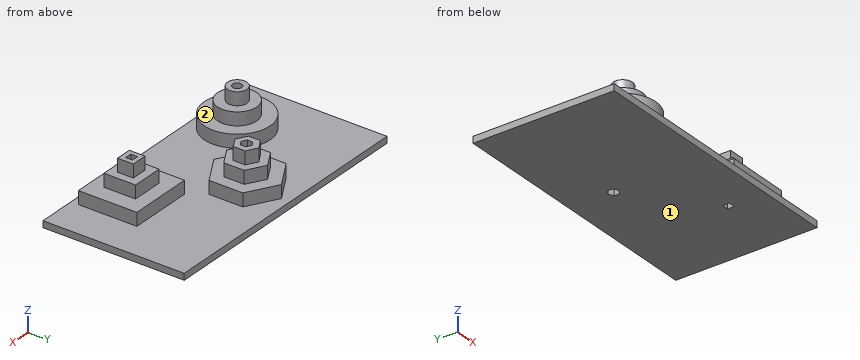
from build123d import *

# Parameters (mm, degrees)
SKETCH_R        = 50.540208
PAD_DEPTH       = 20
SKETCH001_R     = 30.027683
PAD001_DEPTH    = 20
SKETCH002_R     = 15.008606
PAD002_DEPTH    = 20
SKETCH003_R     = 7.050667
POCKET_DEPTH    = 60.001
SKETCH004_W     = 420.746094
SKETCH004_H     = 217.580834
PAD003_DEPTH    = 10
SKETCH005_W     = 98.75679
SKETCH005_H     = 90.115562
PAD004_DEPTH    = 20
SKETCH006_W     = 48.761093
SKETCH006_H     = 48.761156
PAD005_DEPTH    = 20
SKETCH007_W     = 24.319153
SKETCH007_H     = 24.30114
PAD006_DEPTH    = 20
SKETCH008_W     = 10.654495
SKETCH008_H     = 10.502288
POCKET001_DEPTH = 70.001
PAD007_DEPTH    = 20
PAD008_DEPTH    = 20
PAD009_DEPTH    = 20
POCKET002_DEPTH = 70.001


with BuildPart() as part:
    # Sketch → Pad (new body)
    with BuildSketch(Plane.XY):
        Circle(SKETCH_R)
    extrude(amount=PAD_DEPTH)

    # Sketch001 (on Face3 of Pad) → Pad001 (join)
    with BuildSketch(Plane.XY.offset(20)):
        Circle(SKETCH001_R)
    extrude(amount=PAD001_DEPTH)

    # Sketch002 (on Face5 of Pad001) → Pad002 (join)
    with BuildSketch(Plane.XY.offset(40)):
        Circle(SKETCH002_R)
    extrude(amount=PAD002_DEPTH)

    # Sketch003 (on Face7 of Pad002) → Pocket (cut, through all)
    with BuildSketch(Plane.XY.offset(60)):
        Circle(SKETCH003_R)
    extrude(amount=-POCKET_DEPTH, mode=Mode.SUBTRACT)

    # Sketch004 → Pad003 (join)
    with BuildSketch(Plane.XY):
        with Locations((116.873352, 52.568348)):
            Rectangle(SKETCH004_W, SKETCH004_H)
    extrude(amount=-PAD003_DEPTH)

    # Sketch005 (on Face4 of Pad003) → Pad004 (join)
    with BuildSketch(Plane.XY):
        with Locations((219.817588, 0.267387)):
            Rectangle(SKETCH005_W, SKETCH005_H)
    extrude(amount=PAD004_DEPTH)

    # Sketch006 (on Face13 of Pad004) → Pad005 (join)
    with BuildSketch(Plane.XY.offset(20)):
        with Locations((219.351036, -0.022332)):
            Rectangle(SKETCH006_W, SKETCH006_H)
    extrude(amount=PAD005_DEPTH)

    # Sketch007 (on Face20 of Pad005) → Pad006 (join)
    with BuildSketch(Plane.XY.offset(40)):
        with Locations((219.415116, -0.255952)):
            Rectangle(SKETCH007_W, SKETCH007_H)
    extrude(amount=PAD006_DEPTH)

    # Sketch008 (on Face27 of Pad006) → Pocket001 (cut, through all)
    with BuildSketch(Plane.XY.offset(60)):
        with Locations((219.071236, -0.040661)):
            Rectangle(SKETCH008_W, SKETCH008_H)
    extrude(amount=-POCKET001_DEPTH, mode=Mode.SUBTRACT)

    # Sketch009 (on Face4 of Pocket001) → Pad007 (join)
    with BuildSketch(Plane.XY):
        Polygon((152.636142, 69.881975), (152.636142, 121.928939), (107.562149, 147.952421), (62.488156, 121.928939), (62.488156, 69.881975), (107.562149, 43.858493), align=None)
    extrude(amount=PAD007_DEPTH)

    # Sketch010 (on Face24 of Pad007) → Pad008 (join)
    with BuildSketch(Plane.XY.offset(20)):
        Polygon((107.233368, 63.429135), (134.533937, 79.191126), (134.533937, 110.715108), (107.233368, 126.477099), (79.932799, 110.715108), (79.932799, 79.191126), align=None)
    extrude(amount=PAD008_DEPTH)

    # Sketch011 (on Face43 of Pad008) → Pad009 (join)
    with BuildSketch(Plane.XY.offset(40)):
        Polygon((107.227683, 76.060802), (123.144716, 85.250505), (123.144716, 103.629912), (107.227683, 112.819615), (91.31065, 103.629912), (91.31065, 85.250505), align=None)
    extrude(amount=PAD009_DEPTH)

    # Sketch012 (on Face52 of Pad009) → Pocket002 (cut, through all)
    with BuildSketch(Plane.XY.offset(60)):
        Polygon((107.152039, 85.588319), (114.400809, 89.773399), (114.400809, 98.143557), (107.152039, 102.328637), (99.903269, 98.143557), (99.903269, 89.773399), align=None)
    extrude(amount=-POCKET002_DEPTH, mode=Mode.SUBTRACT)


solid = part.part
Check sheet for the modelled part. Datum: model origin and axes. Units: mm. Face numbers are marked on the shaded views. Coordinates: 2 decimals unless noted, no trailing zeros. Loops run counter-clockwise (first coordinate to the right, second up) from the corner with the lowest first, then second, coordinate; pieces in that order, holes last. Notation, with made-up numbers: (10, 65.5) -> (51, 65.5) arc R6 ccw to (51, 71.5) -> close; hole circle Ø11 at (2, 4.25). An arc over 180 degrees is marked (long way). Write item = value, one per line. Start each with the question number.
1. Section check C-C on x = 157. Record the cut outline in (y, z), then the cut area to 3 significant figures.
2. Depth check by flat-ended pin: P1, Ø8, axis at y = 1.5, z = 17.5, coming from the -X side; P2, Ø22, axis at x = 219, z = 51.5, coming from the +Y side; P3, Ø6.5, axis at y = 96, z = 35.5, coming from the +X side. Enter the tip coordinate at first touch or a pass-through.
3. Draft check along X on the marked faces 1 and 2. Enter one of: released by +X, released by -X, zero draft, split by the parting line, or undercut.
4. Section check B-B on x = 0. Record the cut outline in (y, z).
5. Material ranges on line 1 (Y direction, x = 0, z = 14); line 2 (Y direction, x = 0, z = 33.5); line 3 (X direction, y = 45, z = 7) (3 decimals), recorded low to high.
6. Section check A-A on z = 33.5. Record the cut outline in (x, y), then the cut area to 3 significant figures.
Responses:
q1.outline = (-56.22, -10) -> (161.36, -10) -> (161.36, 0) -> (-56.22, 0) -> close
q1.area = 2,180 mm2
q2.P1 = -50.54
q2.P2 = 11.89
q2.P3 = 134.53
q3.face_1 = zero draft
q3.face_2 = undercut
q4.outline = (-56.22, -10) -> (161.36, -10) -> (161.36, 0) -> (50.54, 0) -> (50.54, 20) -> (30.03, 20) -> (30.03, 40) -> (15.01, 40) -> (15.01, 60) -> (7.05, 60) -> (7.05, 0) -> (-7.05, 0) -> (-7.05, 60) -> (-15.01, 60) -> (-15.01, 40) -> (-30.03, 40) -> (-30.03, 20) -> (-50.54, 20) -> (-50.54, 0) -> (-56.22, 0) -> close
q5.line_1 = -50.54 to -7.05, 7.05 to 50.54
q5.line_2 = -30.03 to -7.05, 7.05 to 30.03
q5.line_3 = -23.007 to 23.007, 105.585 to 109.539, 170.439 to 269.196
q6.outline = circle Ø60.06 at (0, 0); (79.93, 79.19) -> (107.23, 63.43) -> (134.53, 79.19) -> (134.53, 110.72) -> (107.23, 126.48) -> (79.93, 110.72) -> close; (194.97, -24.4) -> (243.73, -24.4) -> (243.73, 24.36) -> (194.97, 24.36) -> close; hole circle Ø14.1 at (0, 0); hole (99.9, 89.77) -> (107.15, 85.59) -> (114.4, 89.77) -> (114.4, 98.14) -> (107.15, 102.33) -> (99.9, 98.14) -> close; hole (213.74, -5.29) -> (224.4, -5.29) -> (224.4, 5.21) -> (213.74, 5.21) -> close
q6.area = 7,340 mm2
